Verification items for the finished model (mm, model axes). A direction names the side the tool comes from. Give positions to 0.01 mm unless a question says otherwise; leave off trailing zeros. Loops run counter-clockwise (first coordinate to the right, second up) from the corner with the lowest first, then second, coordinate; pieces in that order, holes last. Notation, with made-up numbers: M 55.5,41 L 66.5,41 A23 cw 66.5,56 Z; hole C 20,-11 d6. An arc over 180 degrees is marked long. Answer in a Markdown table with one row per item.
```python
from build123d import *

# Parameters (mm, degrees)
F1_DEPTH      = 73.914
F1_DEPTH_BACK = 73.914
F2_DEPTH      = 7.9375
F3_DEPTH      = 25.4


with BuildPart() as f1:
    # F0 (on Front) → F1 (new body, two sides)
    with BuildSketch(Plane.XZ) as f1_sk:
        Polygon((-41.275, 9.525), (-41.275, -9.525), (41.275, -9.525), (41.275, 9.525), (22.225, 9.525), align=None)
    extrude(amount=F1_DEPTH)
    extrude(f1_sk.sketch, amount=-F1_DEPTH_BACK)

    # F0 (on Front) → F2 (join, symmetric)
    with BuildSketch(Plane.XZ):
        with BuildLine():
            add(Edge.make_bspline(
                [(-41.275, 9.525), (-40.226812, 42.592709), (20.461641, 48.679743), (55.192691, 49.732862)],
                knots=[0, 0, 0, 0, 104.352522, 104.352522, 104.352522, 104.352522], degree=3))
            Line((-41.275, 9.525), (22.225, 9.525))
            Line((22.225, 9.525), (22.225, 14.862752))
            ThreePointArc((22.225, 14.862752), (31.771716, 38.856466), (55.192691, 49.732862))
        make_face()
    extrude(amount=F2_DEPTH, both=True)

    # F0 (on Front) → F3 (join, symmetric)
    with BuildSketch(Plane.XZ):
        Polygon((89.471519, 49.787752), (70.500782, 49.787752), (70.500782, 30.737752), (89.471519, 30.737752), (95.900782, 30.737752), (95.900782, 49.787752), align=None)
        with BuildLine():
            Line((22.225, 9.525), (41.275, 9.525))
            Line((41.275, 9.525), (41.275, 14.862752))
            ThreePointArc((41.275, 14.862752), (45.92468, 26.088072), (57.15, 30.737752))
            Line((57.15, 30.737752), (70.500782, 30.737752))
            Line((70.500782, 30.737752), (70.500782, 49.787752))
            Line((70.500782, 49.787752), (57.15, 49.787752))
            add(Edge.make_bspline(
                [(55.192691, 49.732862), (55.854758, 49.752937), (56.507392, 49.771183), (57.15, 49.787752)],
                knots=[104.352522, 104.352522, 104.352522, 104.352522, 106.34176, 106.34176, 106.34176, 106.34176], degree=3))
            ThreePointArc((55.192691, 49.732862), (31.771716, 38.856466), (22.225, 14.862752))
            Line((22.225, 14.862752), (22.225, 9.525))
        make_face()
    extrude(amount=F3_DEPTH, both=True)

    # F0 (on Front) → F4 (revolve)
    with BuildSketch(Plane.XZ):
        Polygon((121.300782, 54.816952), (95.900782, 54.816952), (95.900782, 49.787752), (95.900782, 30.737752), (95.900782, 26.241952), (121.300782, 26.241952), align=None)
    revolve(axis=Axis((95.900782, 0, 40.529452), (0, 0, -1)))


solid = f1.part
```
Item 1: Sectioned sample at A-A (x = 78.5). Record the cut outline in (y, z), and give its area (3 significant figures).
Reported:
| item | result |
|---|---|
| outline | M -25.4,30.74 L -18.5,30.74 L -18.5,26.24 L 18.5,26.24 L 18.5,30.74 L 25.4,30.74 L 25.4,49.79 L 18.5,49.79 L 18.5,54.82 L -18.5,54.82 L -18.5,49.79 L -25.4,49.79 Z |
| area | 1,320 mm^2 |
Item 2: Sectioned sample at C-C (y = -36.5). Record the cut outline in (x, z) (3 decimals), and give its area (3 significant figures).
Reported:
| item | result |
|---|---|
| outline | M -41.275,-9.525 L 41.275,-9.525 L 41.275,9.525 L -41.275,9.525 Z |
| area | 1,570 mm^2 |
Item 3: Scan lines: L1, parallel to Z at x = 39.5, y = -45 (3 decimals); L2, parallel to X at y = 26, z = 9 (3 decimals); L3, parallel to Y at x = -34.5, z = 25. Record each from-to range of solid material in increasing order. Write a range as [from, to].
Reported:
| item | result |
|---|---|
| L1 | z = [-9.525, 9.525] |
| L2 | x = [-41.275, 41.275] |
| L3 | y = [-7.94, 7.94] |
Item 4: Release check for a two-part mould opening along X. For faces 6 (the cylindrical face through (32.028, 16.547, 39.124)), 7 (the flat face through (96, 0, 26.242)), 8 (the flat face through (41.275, -1, 0)), 9 (the flat face through (68, 0, 30.738)) record: released by +X, released by -X, zero draft, split by the parting line, or undercut.
Reported:
| item | result |
|---|---|
| face 6 | released by -X |
| face 7 | zero draft |
| face 8 | released by +X |
| face 9 | undercut |
Item 5: Sectioned sample at B-B (z = 3). Record the cut outline in (x, y) (3 decimals), and give its area (3 significant figures).
Reported:
| item | result |
|---|---|
| outline | M -41.275,-73.914 L 41.275,-73.914 L 41.275,73.914 L -41.275,73.914 Z |
| area | 12,200 mm^2 |
Item 6: Tool access check on faces 1 (the cylindrical face through (32.028, -16.791, 39.124)), 2 (the flat face through (59, 25.4, 34)), 3 (the flat face through (22.225, 17, 12)), 4 (the cylindrical face through (45.8, -0.36, 25.96)), 5 (the flat face through (59, -25.4, 34)). Record the directions out of +Z, -Z, +X, -X, +Y, -Y that give a thin tool (end or side, any length) a straight path to the whole face; none if there is none.
Reported:
| item | result |
|---|---|
| face 1 | +Z, -X, -Y |
| face 2 | +Z, +X, -X, +Y |
| face 3 | +Z, -X, +Y |
| face 4 | -Z, +Y, -Y |
| face 5 | +Z, +X, -X, -Y |
Item 7: Go/stop test with flat-tipped pins: pin 1 (19.5 mm diameter, centred on y = -35, z = 4, fed in from +X) (3 decimals); pin 2 (8 mm diameter, centred on y = 12, z = 31, fed in from +X); pin 3 (19.5 mm diameter, centred on x = 71.5, y = 2.5, fed in from -Z). Record where each tip stops, or that it passes through.
Reported:
| item | result |
|---|---|
| pin 1 | stops at x = 41.275 |
| pin 2 | stops at x = 120.01 |
| pin 3 | stops at z = 26.24 |
